Input: part model. Units: mm. Frame: model coordinates. Face numbers are marked on the shaded views. A direction names the side the tool comes from. Round coordinates to 2 decimals unless told otherwise and drop trailing zeros. Loops run counter-clockwise (first coordinate to the right, second up) from the corner with the lowest first, then second, coordinate; pieces in that order, holes last. Notation, with made-up numbers: M 56.25,1 L 99.25,1 A13 ccw 99.25,26 Z; hole C -12,-38 d6. An arc over 180 degrees is marked long. Return JSON: item names as keys, results as strings. Group by question number.
1) Section B-B (x = -84.5). Count the separate pieces of the cut face and the enclosed holes in it, plus the area to 3 significant figures.
2) Material intervals for line 1 (Y direction, x = -83, z = 1.25) (1 decimal); line 2 (X direction, y = 18, z = 1) (3 decimals); line 3 (Y direction, x = -60, z = 2) (3 decimals), sorted ascending. Write a range as from..to.
3) Mould query, pull axis X, two halves, no side actions, for the marked faces 1, 2, 3 and 4. Classes: +X half, -X half, draft (parallel to the pull), parting line (faces both ways), or undercut.
4) Section A-A (y = -23.5). Output: boundary loops of the cut face in (x, z) (3 decimals), plus the area to 3 significant figures.
5) Access query for the marked faces 5 and 6. Directions: +Z, -Z, +X, -X, +Y, -Y. A direction counts if a zero-diameter tool reaches every point of the face in a straight line with its end or side. Return the directions, or none.
6) Contact query for a flat-ended pin moving along its axis: P1, Ø2, axis at x = -100.01, y = -30.16, coming from the +Z side. Output: stop coordinate, or through.
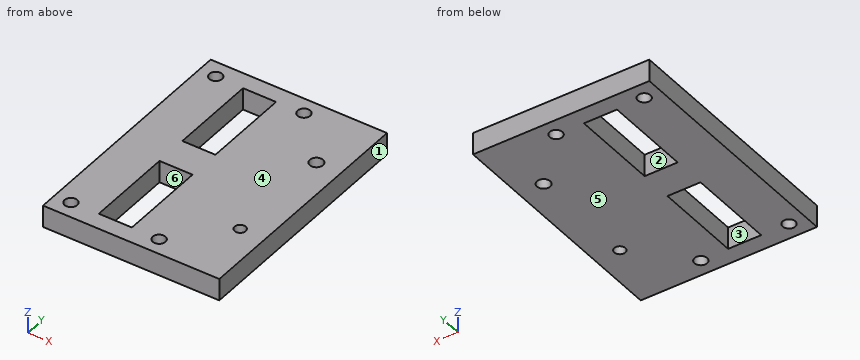
from build123d import *

# Parameters (mm, degrees)
F0_W     = 34.925
F0_H     = 69.85
F0_R     = 1.8288
F0_W_2   = 9.525
F0_H_2   = 25.273
F0_W_3   = 15.875
F0_R_2   = 1.5875
F1_DEPTH = 6.35
F2_D     = 3.6576
F3_D     = 3.7973


# Not quite as in the source:
# - a feature names something its author has since deleted; it is built from what else it names


with BuildPart() as f1:
    # F0 (on Top) → F1 (new body)
    with BuildSketch(Plane.XY):
        with Locations((-87.3125, 0)):
            Rectangle(F0_W, F0_H)
        with Locations((-100.0125, -30.1625)):
            Circle(F0_R, mode=Mode.SUBTRACT)
        with Locations((-87.3125, -17.399)):
            Rectangle(F0_W_2, F0_H_2, mode=Mode.SUBTRACT)
        with Locations((-74.6125, -30.1625)):
            Circle(F0_R, mode=Mode.SUBTRACT)
        with Locations((-87.3125, 17.399)):
            Rectangle(F0_W_2, F0_H_2, mode=Mode.SUBTRACT)
        with Locations((-100.0125, 30.1625)):
            Circle(F0_R, mode=Mode.SUBTRACT)
        with Locations((-74.6125, 30.1625)):
            Circle(F0_R, mode=Mode.SUBTRACT)
        with Locations((-61.9125, 0)):
            Rectangle(F0_W_3, F0_H)
        with Locations((-61.1378, -15.875)):
            Circle(F0_R_2, mode=Mode.SUBTRACT)
        with Locations((-61.1378, 15.875)):
            Circle(F0_R_2, mode=Mode.SUBTRACT)
        with Locations((-100.0125, -30.1625)):
            Circle(F0_R)
        with Locations((-100.0125, 30.1625)):
            Circle(F0_R)
        with Locations((-74.6125, 30.1625)):
            Circle(F0_R)
        with Locations((-74.6125, -30.1625)):
            Circle(F0_R)
        with Locations((-61.1378, 15.875)):
            Circle(F0_R_2)
    extrude(amount=F1_DEPTH)

    # F2 (through all)
    with Locations(Plane(origin=(0, 0, 0), x_dir=(1, 0, 0), z_dir=(0, 0, -1))):
        with Locations((-100.0125, -30.1625), (-74.6125, -30.1625), (-74.6125, 30.1625), (-100.0125, 30.1625)):
            Hole(F2_D / 2)

    # F3 (through all)
    with Locations(Plane(origin=(0, 0, 0), x_dir=(1, 0, 0), z_dir=(0, 0, -1))):
        with Locations((-61.1378, -15.875)):
            Hole(F3_D / 2)


solid = f1.part
Returned:
{
 "1": {"separate pieces": "3", "enclosed holes": "0", "area": "123 mm^2"},
 "2": {"line 1": "y = -34.9..-30, -4.8..4.8, 30..34.9", "line 2": "x = -104.775..-92.075, -82.55..-53.975", "line 3": "y = -34.925..-16.982, -14.768..14.355, 17.395..34.925"},
 "3": {"face 1": "+X half", "face 2": "undercut", "face 3": "undercut", "face 4": "draft"},
 "4": {"outline": "M -104.775,0 L -92.075,0 L -92.075,6.35 L -104.775,6.35 Z; M -82.55,0 L -53.975,0 L -53.975,6.35 L -82.55,6.35 Z", "area": "262 mm^2"},
 "5": {"face 5": "-Z, +X, -X, +Y, -Y", "face 6": "+Z, -Z"},
 "6": {"P1": "passes through"}
}
